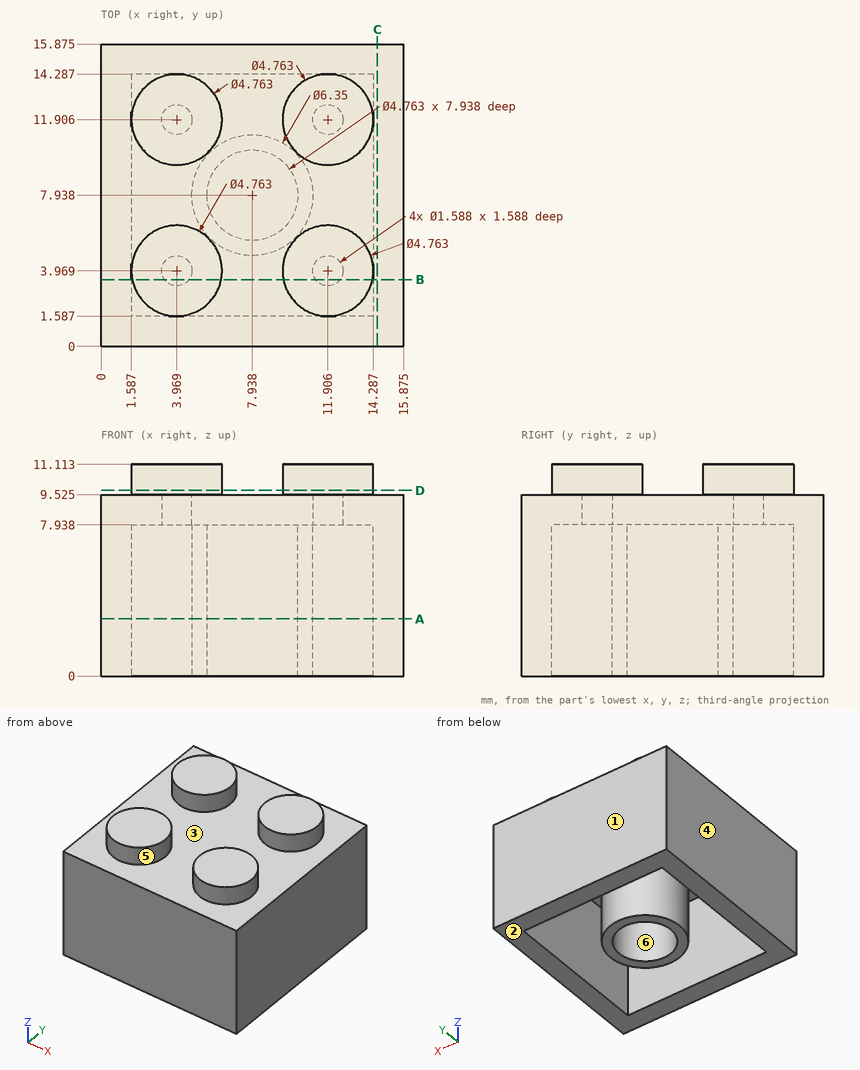
Source: three-view drawing plus pictorial views. Frame: mm from the lowest corner of the part. A direction names the side the tool comes from. Round coordinates to 2 decimals unless told otherwise and drop trailing zeros. Order: outer loops, then holes, each group sorted by start corner. A loop starts at its lowest first (then second) coordinate and runs counter-clockwise, first axis right, second up. Notation, with made-up numbers: (-19, 13.25) -> (13, 13.25) arc R14 cw to (13, 38.25) -> close; hole circle Ø4 at (33.25, 58.5). An arc over 180 degrees is marked (long way). Use one line per item in the form item = value. Start each with the question number.
1. Cut plane A-A (z = 3). Count the separate pieces of the cut face and the enclosed holes in it.
2. Pin query (flat end, axial travel): pin 1 Ø1 at (x, y) = (11.91, 11.91) entering from -Z (1 decimal); pin 2 Ø3 at (x, y) = (7.94, 7.94) entering from +Z (1 decimal); pin 3 Ø1.7 at (x, y) = (11.5, 3.5) entering from -Z. Return the tip coordinate at first contact, or that it passes through.
3. Cut plane C-C (x = 14.5). Return the cut outline in (y, z) (1 decimal).
4. Line query: probe 1 along Y at (x, z) = (14, 6) (1 decimal); probe 2 along Y at (x, z) = (9, 4.5) (1 decimal). Output: solid intervals per line, ascending.
5. Cut plane D-D (z = 9.75). Return the cut outline in (x, y).
6. Cut plane B-B (y = 3.5). Return the cut outline in (x, z) (1 decimal).
7. Reachability of the marked faces 4, 5 and 6 from +Z, -Z, +X, -X, +Y, -Y: full face, straight path, thin tool, end or side. Return the list, or none.
8. Draft query along Y for the marked faces 1, 2 and 3. Return one class per face: pulls with the +Y half, pulls with the -Y half, needs draft (parallel to the pull), parting line crosses it, or undercut.
Solution:
q1.separate_pieces = 2
q1.enclosed_holes = 2
q2.pin_1 = 9.5
q2.pin_2 = 9.5
q2.pin_3 = 7.94
q3.outline = (0, 0) -> (15.9, 0) -> (15.9, 9.5) -> (0, 9.5) -> close
q4.probe_1 = 0 to 1.6, 14.3 to 15.9
q4.probe_2 = 0 to 1.6, 4.9 to 5.8, 10.1 to 10.9, 14.3 to 15.9
q5.outline = circle Ø4.76 at (3.97, 3.97); circle Ø4.76 at (3.97, 11.91); circle Ø4.76 at (11.91, 3.97); circle Ø4.76 at (11.91, 11.91)
q6.outline = (0, 0) -> (1.6, 0) -> (1.6, 7.9) -> (3.3, 7.9) -> (3.3, 9.5) -> (4.6, 9.5) -> (4.6, 7.9) -> (11.3, 7.9) -> (11.3, 9.5) -> (12.5, 9.5) -> (12.5, 7.9) -> (14.3, 7.9) -> (14.3, 0) -> (15.9, 0) -> (15.9, 9.5) -> (14.2, 9.5) -> (14.2, 11.1) -> (9.6, 11.1) -> (9.6, 9.5) -> (6.3, 9.5) -> (6.3, 11.1) -> (1.6, 11.1) -> (1.6, 9.5) -> (0, 9.5) -> close
q7.face_4 = +Z, -Z, -X, +Y, -Y
q7.face_5 = +Z
q7.face_6 = -Z
q8.face_1 = pulls with the +Y half
q8.face_2 = needs draft
q8.face_3 = undercut
